Autodesk Inventor part; units mm, degrees
ref_plane "YZ Plane" through (0, 0, 0) normal (1, 0, 0) x (0, 1, 0)
ref_plane "XZ Plane" through (0, 0, 0) normal (0, 1, 0) x (-1, 0, 0)
ref_plane "XY Plane" through (0, 0, 0) normal (0, 0, 1) x (1, 0, 0)
sketch "Sketch1" plane through (0, 0, 0) normal (0, 1, 0) x (-1, 0, 0)
  line L0 (0, 0) -> (-10, 0)
  line L1 (-10, 0) -> (-10, -10)
  line L2 (-10, -10) -> (0, -10)
  line L3 (0, -10) -> (0, 0)
  dimension "d0" = 10
  dimension "d1" = 10
extrude "Extrusion1" add sketch "Sketch1" along normal blind 10
sketch "Sketch2" plane through (0, 10, 0) normal (0, 1, 0) x (1, 0, 0)
  line L0 (0, 10) -> (0, 0)
  line L1 (10, 0) -> (10, 10)
  line L2 (0, 0) -> (10, 10)
  line L3 (10, 10) -> (0, 10)
  line L4 (10, 0) -> (0, 10)
  line L5 (5, 5) -> (7.1771, 5)
sketch "Sketch3" plane through (0, 10, 0) normal (0, 1, 0) x (1, 0, 0)
  point P0 (0, 0)
hole "Hole1" at (5, 10, -5) direction (0, -1, 0) diameter 3.2 end through all
properties part number "distanziale cella di carico"
Build history of the part. All positions in model axes, mm. Give positions to 0.01 mm unless a question says otherwise; leave off trailing zeros. Order: outer loops, then holes, each group sorted by start corner. A loop starts at its lowest first (then second) coordinate and runs counter-clockwise, first axis right, second up. Notation, with made-up numbers: M 35.25,37 L 76.25,37 A32 ccw 76.25,66 Z; hole C -30.75,7 d11. An arc over 180 degrees is marked long. Put each result on its own line as item: value.
Item 1: Cut at A-A on z = -5. Write the cut outline in (x, y).
Results are:
outline: M 0,0 L 3.4,0 L 3.4,10 L 0,10 Z; M 6.6,0 L 10,0 L 10,10 L 6.6,10 Z
Item 2: Wall check: probe 1 along X at (y, z) = (5, -5); probe 2 along Z at (x, y) = (5, 6); probe 3 along X at (y, z) = (6.75, -5.75). Give the ranges that are in metal, low to high.
Results are:
probe 1: 0 to 3.4, 6.6 to 10
probe 2: -10 to -6.6, -3.4 to 0
probe 3: 0 to 3.59, 6.41 to 10
Item 3: Pull direction Z, two halves, no side cores. Call faces 1 (the face through (5, 5, 0)), 2 (the face through (5, 0, -3)), 3 (the face through (4.93, 4.93, -6.6)), 4 (the face through (5, 5, -10)): +Z half, -Z half, draft (parallel to the pull), parting line (faces both ways), or undercut.
Results are:
face 1: +Z half
face 2: draft
face 3: undercut
face 4: -Z half
Item 4: Cut at C-C on x = 5. Write the cut outline in (y, z).
Results are:
outline: M 0,-10 L 10,-10 L 10,-6.6 L 0,-6.6 Z; M 0,-3.4 L 10,-3.4 L 10,0 L 0,0 Z
Item 5: Cut at B-B on y = 6.5. Write the cut outline in (x, z), then the cut area to 3 significant figures.
Results are:
outline: M 0,-10 L 10,-10 L 10,0 L 0,0 Z; hole C 5,-5 d3.2
area: 92.0 mm2
